Verification items for the finished model (mm, model axes). A direction names the side the tool comes from. Coordinates: 2 decimals unless noted, no trailing zeros. Order: outer loops, then holes, each group sorted by start corner. A loop starts at its lowest first (then second) coordinate and runs counter-clockwise, first axis right, second up.
Q1. Cross-section at B-B, the plane z = -3. Record the boundary of the cut face in (x, y).
Q2. Draft check along Z on faces 4 (the conical face through (-13.878, 23.791, 23.723)), 5 (the flat face through (0, -26, 20)), 6 (the cylindrical face through (-18.2, 13.9, 15.2)). Enter one of: pulls with the +Z half, pulls with the -Z half, needs draft (parallel to the pull), parting line crosses it, or undercut.
Q3. Depth check by flat-ended pin: P1, Ø6, axis at y = -5, z = 7.5, coming from the -X side; P2, Ø6, axis at y = -8, z = 19, coming from the -X side; P3, Ø3, axis at y = -0.5, z = 12, coming from the -X side. Enter the tip coordinate at first touch or a pass-through.
Q4. Thickness scan on line 1 (Z direction, x = -18, y = -19.5); line 2 (Z direction, x = 23, y = 4); line 3 (X direction, y = 11, z = 8.5). Record the ranges inside material, lowest first.
Q5. Cross-section at A-A, the plane x = 0. Record the boundary of the cut face in (y, z), and give its area (3 significant figures).
Q6. Set-up check for faces 1 (the flat face through (0, 0, 23.988)), 2 (the cylindrical face through (-17.62, -16.15, -0.18)), 3 (the flat face through (20, 12, 16.388)): record each of +Z, -Z, +X, -X, +Y, -Y from which the full face is reachable in a straight line by a thin tool's end or side.
Q7. Cross-section at C-C, the plane z = 15.5. Record the boundary of the cut face in (x, y).
Autodesk Inventor part; units mm, degrees
ref_plane "YZ Plane" through (0, 0, 0) normal (1, 0, 0) x (0, 1, 0)
ref_plane "XZ Plane" through (0, 0, 0) normal (0, 1, 0) x (-1, 0, 0)
ref_plane "XY Plane" through (0, 0, 0) normal (0, 0, 1) x (1, 0, 0)
sketch "Szkic7" plane through (0, 0, 0) normal (0, 0, 1) x (1, 0, 0)
  circle A0 centre (0, 0) radius 23.9015
  dimension "d35" = 47.803
extrude "Wyciągnięcie proste2" add sketch "Szkic7" along normal mid plane 28.025
chamfer "Faza2" distance 1 angle 45 1 edges at (-23.9015, 0, 14.0125)
sketch "Szkic9" plane through (0, 0, 14.0125) normal (0, 0, 1) x (1, 0, 0)
  circle A0 centre (0, 0) radius 22.9015
extrude "Wyciągnięcie proste3" add sketch "Szkic9" along normal blind 2.375
sketch "Szkic10" plane through (0, 0, 16.3875) normal (0, 0, 1) x (1, 0, 0)
  line L0 (-15.0111, 26) -> (15.0111, 26)
  line L1 (15.0111, 26) -> (30.0222, 0)
  line L2 (30.0222, 0) -> (15.0111, -26)
  line L3 (15.0111, -26) -> (-15.0111, -26)
  line L4 (-15.0111, -26) -> (-30.0222, 0)
  line L5 (-30.0222, 0) -> (-15.0111, 26)
  line L6 (0, 33.4621) -> (0, -33.4621) construction
  line L7 (-33.4621, 0) -> (33.4621, 0) construction
  point P0 (0, 0)
  point P1 (0, 0)
  point P2 (0, 26)
  dimension "d44" = 52
extrude "Wyciągnięcie proste4" add sketch "Szkic10" along normal blind 7.6
sketch "Szkic12" plane through (0, 0, 0) normal (0, 1, 0) x (-1, 0, 0)
  line L0 (0, -2.1463) -> (0, 12.8775) construction
  line L1 (-15.0111, 16.3875) -> (-15.0111, 23.9875) construction
  line L2 (-30.0222, 23.9875) -> (-15.0111, 23.9875) construction
  line L3 (-30.0222, 16.3875) -> (-30.0222, 23.9875)
  line L4 (-30.0222, 23.0586) -> (-26.5555, 23.9875)
  line L5 (-30.0222, 23.9875) -> (-15.0111, 23.9875)
  line L6 (-30.0222, 16.3875) -> (-15.0111, 16.3875)
  point P0 (0, 0)
  dimension "d50" = 15
  dimension "d51" = 3.4667
revolve "Obrót2" cut sketch "Szkic12" angle 360 about axis through (0, 0, -10) along (0, 0, 1)
thread "Gwint3"
chamfer "Faza3" distance 1 angle 45 1 edges at (-23.9015, 0, -14.0125)
equation "\"d35\" = OD"
equation "\"d36\" = 0.7375 * L"
equation "\"d42\" = 0.0625 * L"
equation "\"d44\" = SW"
equation "\"d45\" = 0.2 * L"
equation "\"d51\" = 0.0666667 * SW"
equation "\"SzerokośćGięciaPodcięcia\" = Grubość"
equation "\"RozmiarPodcięciaNarożnika\" = 4 * Grubość"
equation "\"PromieńPrzejścia\" = PromieńGięcia"
equation "\"Rozmiar_promienia_Jacobiego\" = PromieńGięcia"
equation "\"Wielk_odstępu\" = Grubość"
equation "\"d2\" = PromieńGięcia"
equation "\"d23\" = PromieńGięcia"
equation "\"OD\" = 47.803"
equation "\"SW\" = 52"
equation "\"L\" = 38"
properties part number "Korek sześciokątny BSP 1 1/2'' L=38" material "304"
Check values:
1. outline: circle Ø47.8 at (0, 0)
2. face 4: pulls with the +Z half
2. face 5: needs draft
2. face 6: undercut
3. P1: stops at x = -23.82
3. P2: stops at x = -27.14
3. P3: stops at x = -23.9
4. line 1: z = 16.39 to 23.99
4. line 2: z = -13.57 to 13.57, 16.39 to 23.99
4. line 3: x = -21.22 to 21.22
5. outline: (-26, 16.39) - (-22.9, 16.39) - (-22.9, 14.01) - (-23.9, 13.01) - (-23.9, -13.01) - (-22.9, -14.01) - (22.9, -14.01) - (23.9, -13.01) - (23.9, 13.01) - (22.9, 14.01) - (22.9, 16.39) - (26, 16.39) - (26, 23.99) - (-26, 23.99) - close
5. area: 1,840 mm2
6. face 1: +Z, +X, -X, +Y, -Y
6. face 2: -Z
6. face 3: none
7. outline: circle Ø45.8 at (0, 0)
